```python
from build123d import *

# Parameters (mm, degrees)
SKETCH2_W           = 40
SKETCH2_H           = 500
BOSS_EXTRUDE1_DEPTH = 40
SKETCH3_W           = 15
SKETCH3_H           = 23
SKETCH3_H_2         = 15
SKETCH3_W_2         = 23
CUT_EXTRUDE1_DEPTH  = 1000
CUT_EXTRUDE2_DEPTH  = 1000


with BuildPart() as part:
    # Sketch2 → Boss-Extrude1 (new body)
    with BuildSketch(Plane.XY):
        with Locations((-324.597701149, 61.781609195)):
            Rectangle(SKETCH2_W, SKETCH2_H)
    extrude(amount=BOSS_EXTRUDE1_DEPTH)

    # Sketch3 → Cut-Extrude1 (cut)
    with BuildSketch(Plane(origin=(0, 311.781609195, 0), x_dir=(1, 0, 0), z_dir=(0, 1, 0))):
        with Locations((-312.097701149, -13.5)):
            Rectangle(SKETCH3_W, SKETCH3_H)
        with Locations((-312.097701149, -32.5)):
            Rectangle(SKETCH3_W, SKETCH3_H_2)
        with Locations((-331.097701149, -32.5)):
            Rectangle(SKETCH3_W_2, SKETCH3_H_2)
    extrude(amount=-CUT_EXTRUDE1_DEPTH, mode=Mode.SUBTRACT)

    # Sketch4 → Cut-Extrude2 (cut)
    with BuildSketch(Plane(origin=(0, 0, 0), x_dir=(-1, 0, 0), z_dir=(0, 0, -1))):
        Polygon((304.597701149, 311.781609195), (344.597701149, 311.781609195), (304.597701149, 271.781609195), align=None)
        Polygon((344.597701149, -188.218390805), (304.597701149, -188.218390805), (304.597701149, -148.218390805), align=None)
    extrude(amount=-CUT_EXTRUDE2_DEPTH, mode=Mode.SUBTRACT)


solid = part.part
```
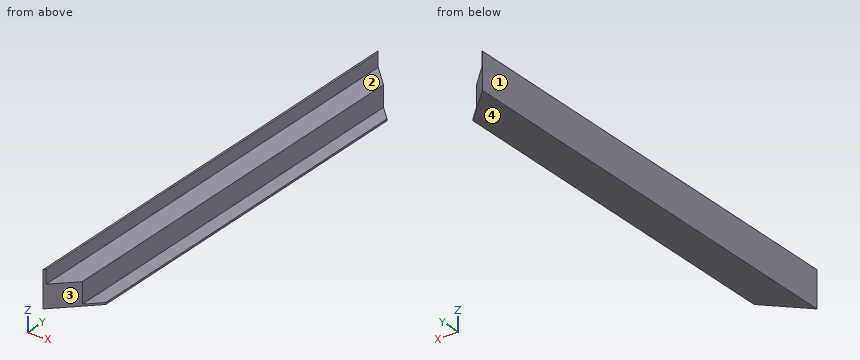
Here's how the part is built. I have some questions about the finished solid (model axes, mm). Face numbers are marked on the shaded views. A direction names the side the tool comes from. Give positions to 0.01 mm unless a question says otherwise; leave off trailing zeros. Write each loop counter-clockwise with the first axis right and the second up, starting at its lowest first coordinate (ties: lowest second). Pieces come first, ordered by that corner, then holes. Notation, with made-up numbers: M 34.25,64.5 L 86.25,64.5 A20 ccw 86.25,71.5 Z; hole C 45.25,52.5 d11. An arc over 180 degrees is marked long. Put each result on its own line as item: value. Start each with the question number.
Item 1: If we section it at B-B, the plane z = 16: Write out the boundary of the cut face in (x, y).
Item 2: I need wall thicknesses on L1, parallel to X at y = 45, z = 26.5; L2, parallel to Z at x = -308, y = 216; L3, parallel to X at y = -95, z = 15.5. Which ranges of each line are inside material? Lowest first, please. Write a range as from..to.
Item 3: On a 3-axis mill with a long thin cutter (end or side, diameter ignored), from which of +Z, -Z, +X, -X, +Y, -Y can I reach the whole of each face in a straight line? I mean the marked faces 1 and 2. Say none if no direction works.
Item 4: If we section it at A-A, the plane y = 231: Write out the boundary of the cut face in (x, z), then the cut area to 3 significant figures.
Item 5: If we section it at C-C, the plane x = -333: Write out the boundary of the cut face in (y, z), then the cut area to 3 significant figures.
Item 6: Thinking about a two-plate mould opening in Y: for the marked faces 3 and 4, which applies, +Y half, -Y half, draft (parallel to the pull), parting line (faces both ways), or undercut?
Item 7: Will these pins go through, and if not, where does the flat tip stop? pin 1 (12 mm diameter, centred on x = -321, z = 16, fed in from -Y); pin 2 (12 mm diameter, centred on y = -43, z = 34, fed in from +X); pin 3 (8 mm diameter, centred on x = -339, y = -18, fed in from +Z); pin 4 (8 mm diameter, centred on x = -322.5, y = -108.5, fed in from +Z).
Values:
1. outline: M -344.6,-188.22 L -319.6,-163.22 L -319.6,286.78 L -344.6,311.78 Z
2. L1: -344.6..-342.6
2. L2: 0..2
2. L3: -344.6..-319.6
3. face 1: +Z, -Z, -X, +Y, -Y
3. face 2: +Z, +X, +Y, -Y
4. outline: M -344.6,0 L -304.6,0 L -304.6,2 L -319.6,2 L -319.6,25 L -342.6,25 L -342.6,40 L -344.6,40 Z
4. area: 685 mm²
5. outline: M -176.62,0 L 300.18,0 L 300.18,25 L -176.62,25 Z
5. area: 11,900 mm²
6. face 3: -Y half
6. face 4: draft
7. pin 1: y = -170.62
7. pin 2: x = -342.6
7. pin 3: z = 40
7. pin 4: z = 25
